from build123d import *

# Parameters (mm, degrees)
ESQUISSE1_R                  = 34.75
ESQUISSE1_R_2                = 32.75
BOSS_EXTRU_1_DEPTH           = 9.4
ESQUISSE2_R                  = 34.75
BOSS_EXTRU_2_DEPTH           = 2
ESQUISSE3_W                  = 1
ESQUISSE3_H                  = 2.5
ENL_V_MAT_EXTRU_1_DEPTH      = 1
ENL_V_MAT_EXTRU_2_DEPTH      = 1.5
ENL_V_MAT_EXTRU_3_DEPTH      = 2
ESQUISSE6_W                  = 3
ESQUISSE6_H                  = 2.5
ENL_V_MAT_EXTRU_4_DEPTH      = 3
ENL_V_MAT_EXTRU_5_DEPTH      = 4
ENL_V_MAT_EXTRU_6_DEPTH      = 5
ENL_V_MAT_EXTRU_7_DEPTH      = 50.697937583
ENL_V_MAT_EXTRU_7_DEPTH_BACK = 50.697937583
ESQUISSE9_R                  = 17.5


with BuildPart() as part:
    # Esquisse1 → Boss.-Extru.1 (new body)
    with BuildSketch(Plane.XY):
        Circle(ESQUISSE1_R)
        Circle(ESQUISSE1_R_2, mode=Mode.SUBTRACT)
    extrude(amount=BOSS_EXTRU_1_DEPTH)

    # Esquisse2 → Boss.-Extru.2 (add)
    with BuildSketch(Plane(origin=(0, 0, 0), x_dir=(-1, 0, 0), z_dir=(0, 0, -1))):
        with Locations(Location((0, 0, 0), (0, 0, 180))):
            Circle(ESQUISSE2_R)
    extrude(amount=-BOSS_EXTRU_2_DEPTH)

    # Esquisse3 → Enlèv. mat.-Extru.1 (cut)
    with BuildSketch(Plane.XY.offset(9.4)):
        with Locations((0, -33.996182984)):
            Rectangle(ESQUISSE3_W, ESQUISSE3_H)
    extrude(amount=-ENL_V_MAT_EXTRU_1_DEPTH, mode=Mode.SUBTRACT)

    # Esquisse4 → Enlèv. mat.-Extru.2 (cut)
    with BuildSketch(Plane.XY.offset(9.4)):
        Polygon((28.729893758, -15.721186491), (27.979893758, -17.020224597), (30.144957267, -18.270224597), (30.894957267, -16.971186491), align=None)
    extrude(amount=-ENL_V_MAT_EXTRU_2_DEPTH, mode=Mode.SUBTRACT)

    # Esquisse5 → Enlèv. mat.-Extru.3 (cut)
    with BuildSketch(Plane.XY.offset(9.4)):
        Polygon((27.849107129, 17.233390036), (28.849107129, 15.501339228), (31.014170638, 16.751339228), (30.014170638, 18.483390036), align=None)
    extrude(amount=-ENL_V_MAT_EXTRU_3_DEPTH, mode=Mode.SUBTRACT)

    # Esquisse6 → Enlèv. mat.-Extru.4 (cut)
    with BuildSketch(Plane.XY.offset(9.4)):
        with Locations((0, 33.965630821)):
            Rectangle(ESQUISSE6_W, ESQUISSE6_H)
    extrude(amount=-ENL_V_MAT_EXTRU_4_DEPTH, mode=Mode.SUBTRACT)

    # Esquisse7 → Enlèv. mat.-Extru.5 (cut)
    with BuildSketch(Plane.XY.offset(9.4)):
        Polygon((-29.309395525, 14.612386319), (-27.309395525, 18.076487935), (-29.474459035, 19.326487935), (-31.474459035, 15.862386319), align=None)
    extrude(amount=-ENL_V_MAT_EXTRU_5_DEPTH, mode=Mode.SUBTRACT)

    # Esquisse8 → Enlèv. mat.-Extru.6 (cut)
    with BuildSketch(Plane.XY.offset(9.4)):
        Polygon((-27.029575227, -18.492283879), (-29.529575227, -14.16215686), (-31.694638736, -15.41215686), (-29.194638736, -19.742283879), align=None)
    extrude(amount=-ENL_V_MAT_EXTRU_6_DEPTH, mode=Mode.SUBTRACT)

    # Esquisse9 → Enlèv. mat.-Extru.7 (cut, two sides: drawn at the far end of the back side and taken through both)
    with BuildSketch(Plane.XY.offset(2).offset(-ENL_V_MAT_EXTRU_7_DEPTH_BACK)):
        Circle(ESQUISSE9_R)
    extrude(amount=ENL_V_MAT_EXTRU_7_DEPTH + ENL_V_MAT_EXTRU_7_DEPTH_BACK, mode=Mode.SUBTRACT)


solid = part.part
Here's how the part is built. I have some questions about the finished solid (model axes, mm). A direction names the side the tool comes from. Give positions to 0.01 mm unless a question says otherwise; leave off trailing zeros. Order: outer loops, then holes, each group sorted by start corner. A loop starts at its lowest first (then second) coordinate and runs counter-clockwise, first axis right, second up. Notation, with made-up numbers: (-11.75, -26) -> (-7.75, -26) arc R27 cw to (-7.75, 2) -> close; hole circle Ø4 at (37.5, -11.5). An arc over 180 degrees is marked (long way). One line per item, written item: value. Start each with the question number.
1. I need wall thicknesses on probe 1 along X at (y, z) = (0, 7); probe 2 along X at (y, z) = (0, 0.5). Which ranges of each line are inside material? Lowest first, please. Write a range as from..to.
2. For faces 1 (the face through (-30.19, 15.12, 7.43)), 2 (the face through (-27.91, -19, 6.94)), 3 (the face through (28.73, 17.74, 8.41)), 4 (the face through (29, -17, 7.9)), which set-ups out of +Z, -Z, +X, -X, +Y, -Y let a thin tool reach every point of the face, with its end or its side?
3. Imagine slicing it at B-B, the plane x = 13. List the corners of the cut face in (y, z) for me, plus the area to 3 significant figures.
4. Will these pins go through, and if not, where does the flat tip stop? pin 1 Ø1 at (y, z) = (-26, 4) entering from -X; pin 2 Ø3.5 at (x, y) = (-29.5, -16.5) entering from +Z; pin 3 Ø3 at (x, y) = (-9, 15) entering from +Z.
5. Imagine slicing it at C-C, the plane y = -30. List the corners of the cut face in (x, z) for me, plus the area to 3 significant figures.
6. We'd pull the mould along X, two halves only. Please class faces 5 (the face through (-16, 29, 9.4)), 6 (the face through (18.68, 29.3, 4.63)), 7 (the face through (-30.39, -14.66, 6.94)): released by +X, released by -X, zero draft, split by the parting line, or undercut.
7. Imagine slicing it at A-A, the plane y = 0. List the corners of the cut face in (x, z) for me.
Values follow:
1. probe 1: x = -34.75..-32.75, 32.75..34.75
1. probe 2: x = -34.75..-17.5, 17.5..34.75
2. face 1: +Z, +Y
2. face 2: +Z, -X
2. face 3: +Z, +X
2. face 4: +Z
3. outline: (-32.23, 0) -> (-11.72, 0) -> (-11.72, 2) -> (-30.06, 2) -> (-30.06, 9.4) -> (-32.23, 9.4) -> close; (11.72, 0) -> (32.23, 0) -> (32.23, 9.4) -> (30.06, 9.4) -> (30.06, 2) -> (11.72, 2) -> close
3. area: 114 mm2
4. pin 1: stops at x = -23.61
4. pin 2: stops at z = 4.4
4. pin 3: stops at z = 2
5. outline: (-17.54, 0) -> (17.54, 0) -> (17.54, 9.4) -> (13.14, 9.4) -> (13.14, 2) -> (-13.14, 2) -> (-13.14, 9.4) -> (-17.54, 9.4) -> close
5. area: 135 mm2
6. face 5: zero draft
6. face 6: split by the parting line
6. face 7: undercut
7. outline: (-34.75, 0) -> (-17.5, 0) -> (-17.5, 2) -> (-32.75, 2) -> (-32.75, 9.4) -> (-34.75, 9.4) -> close; (17.5, 0) -> (34.75, 0) -> (34.75, 9.4) -> (32.75, 9.4) -> (32.75, 2) -> (17.5, 2) -> close
